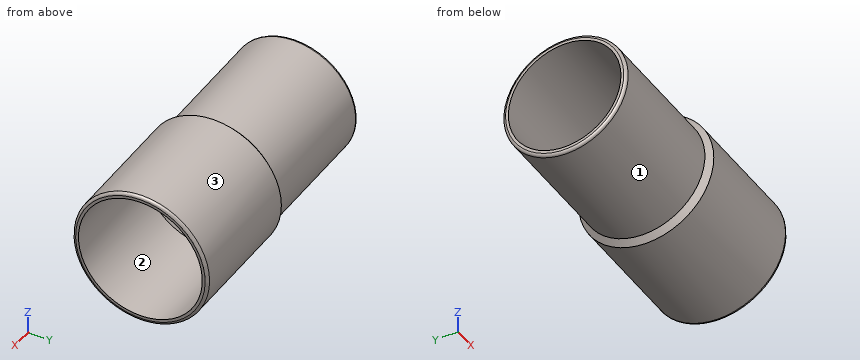
from build123d import *

# Parameters (mm, degrees)
F2_SIZE = 1.99999
F3_R    = 1


# Not quite as in the source:
# - a fillet or chamfer is up to 0.001 mm smaller than in the source, because OpenCascade refuses the exact size


with BuildPart() as f1:
    # F0 (on Front) → F1 (revolve)
    with BuildSketch(Plane.XZ):
        Polygon((-45, 22), (-95, 22), (-95, 20), (-41.2017212381, 20), (-40, 22), (0, 22), (0, 24), (-45, 24), align=None)
    revolve(axis=Axis((-59.3267625081, 0, 0), (-1, 0, 0)))

    # F2 (size 2 in the source; OpenCascade refuses exactly that, so slightly less here)
    f2_edges = [f1.edges().sort_by_distance(p)[0] for p in [
        (-45, 0, -22),
    ]]
    chamfer(f2_edges, length=F2_SIZE)

    # F3
    f3_edges = [f1.edges().sort_by_distance(p)[0] for p in [
        (0, 0, -24),
        (-95, 0, -22),
    ]]
    fillet(f3_edges, radius=F3_R)


solid = f1.part
Design review of the part built by this model. Coordinates are the model's own, in mm. Face numbers are marked on the shaded views. A direction names the side the tool comes from. Round coordinates to 2 decimals unless told otherwise and drop trailing zeros. Write each loop counter-clockwise with the first axis right and the second up, starting at its lowest first coordinate (ties: lowest second). Pieces come first, ordered by that corner, then holes.
Item 1: Consider section D-D on x = -29.5. Give the boundary of the cut face in (y, z), and give its area (3 significant figures).
Item 2: Consider section C-C on x = -66. Give the boundary of the cut face in (y, z).
Item 3: For the marked faces 1, 2 and 3, list the 3-axis set-ups (+Z, -Z, +X, -X, +Y, -Y) from which the entire face can be reached by the end or side of a thin tool; tool diameter is ignored.
Item 4: For pin 1 Ø2 at (x, y) = (-23.5, 12.5) entering from +Z; pin 2 Ø4 at (x, y) = (-71.5, 5.5) entering from -Z; pin 3 Ø8 at (x, y) = (-16, 17) entering from -Z, all flat-tipped, find the tip position at first contact; note any pin that passes through.
Item 5: Wall thickness on L1, parallel to Y at x = -28.5, z = 0; L2, parallel to Y at x = -57, z = 0; L3, parallel to Z at x = -35, y = 0.5: over which ranges is each line inside the solid? List them lowest first.
Check values:
1. outline: circle Ø48 at (0, 0); hole circle Ø44 at (0, 0)
1. area: 289 mm2
2. outline: circle Ø44 at (0, 0); hole circle Ø40 at (0, 0)
3. face 1: -X
3. face 2: +X
3. face 3: +X, -X
4. pin 1: stops at z = 21.07
4. pin 2: stops at z = -21.72
4. pin 3: stops at z = -20.17
5. L1: y = -24 to -22, 22 to 24
5. L2: y = -22 to -20, 20 to 22
5. L3: z = -23.99 to -21.99, 21.99 to 23.99
